from build123d import *

# Parameters (mm, degrees)
SKETCH2_W           = 42
SKETCH2_H           = 42
BOSS_EXTRUDE1_DEPTH = 100
SKETCH3_W           = 10.5
SKETCH3_H           = 42
BOSS_EXTRUDE2_DEPTH = 22
BOSS_EXTRUDE3_DEPTH = 10.5
BOSS_EXTRUDE4_START = -10.5
BOSS_EXTRUDE4_DEPTH = 10.5
SKETCH6_W           = 32
SKETCH6_H           = 32
CUT_EXTRUDE1_DEPTH  = 27
SKETCH7_R           = 3.95
CUT_EXTRUDE2_DEPTH  = 107.92637654
SKETCH9_R           = 3.95
CUT_EXTRUDE3_DEPTH  = 107.92637654
CUT_EXTRUDE4_DEPTH  = 21
FILLET1_R           = 5


with BuildPart() as part:
    # Sketch2 → Boss-Extrude1 (new body)
    with BuildSketch(Plane.XY):
        Rectangle(SKETCH2_W, SKETCH2_H)
    extrude(amount=BOSS_EXTRUDE1_DEPTH)

    # Sketch3 → Boss-Extrude2 (add)
    with BuildSketch(Plane(origin=(0, 0, 0), x_dir=(-1, 0, 0), z_dir=(0, 0, -1))):
        with Locations((15.75, 0)):
            Rectangle(SKETCH3_W, SKETCH3_H)
        with Locations((-15.75, 0)):
            Rectangle(SKETCH3_W, SKETCH3_H)
    extrude(amount=BOSS_EXTRUDE2_DEPTH)

    # Sketch4 → Boss-Extrude3 (add)
    with BuildSketch(Plane.ZY.offset(21)):
        with BuildLine():
            Line((-22, -21), (-22, 21))
            ThreePointArc((-22, 21), (-43, 0), (-22, -21))
        make_face()
    extrude(amount=-BOSS_EXTRUDE3_DEPTH)

    # Sketch5 → Boss-Extrude4 (add)
    with BuildSketch(Plane(origin=(21, 0, 0), x_dir=(0, 0, -1), z_dir=(1, 0, 0)).offset(BOSS_EXTRUDE4_START)):
        with BuildLine():
            Line((22, 21), (22, -21))
            ThreePointArc((22, -21), (43, 0), (22, 21))
        make_face()
    extrude(amount=BOSS_EXTRUDE4_DEPTH)

    # Sketch6 → Cut-Extrude1 (cut)
    with BuildSketch(Plane.XY.offset(100)):
        Rectangle(SKETCH6_W, SKETCH6_H)
    extrude(amount=-CUT_EXTRUDE1_DEPTH, mode=Mode.SUBTRACT)

    # Sketch7 → Cut-Extrude2 (cut, through all)
    with BuildSketch(Plane.ZY.offset(-10.5)):
        with Locations((-22, 0)):
            Circle(SKETCH7_R)
    extrude(amount=-CUT_EXTRUDE2_DEPTH, mode=Mode.SUBTRACT)

    # Sketch9 → Cut-Extrude3 (cut, through all)
    with BuildSketch(Plane(origin=(-10.5, 0, 0), x_dir=(0, 0, -1), z_dir=(1, 0, 0))):
        with Locations(Location((24, 0, 0), (0, 0, 90))):
            Circle(SKETCH9_R)
    extrude(amount=-CUT_EXTRUDE3_DEPTH, mode=Mode.SUBTRACT)

    # Sketch11 → Cut-Extrude4 (cut)
    with BuildSketch(Plane.ZY.offset(-10.5)):
        Polygon((0, 21), (0, 0), (29.025198915, 21), align=None)
        Polygon((29.025198915, -21), (0, 0), (0, -21), align=None)
    extrude(amount=CUT_EXTRUDE4_DEPTH, mode=Mode.SUBTRACT)

    # Fillet1
    fillet1_edges = [part.edges().sort_by_distance(p)[0] for p in [
        (0, 0, 0),
    ]]
    fillet(fillet1_edges, radius=FILLET1_R)


solid = part.part
For this review, take the finished solid that the model builds, in its own axes (mm). A direction names the side the tool comes from. Round coordinates to 2 decimals unless told otherwise and drop trailing zeros. Write each loop counter-clockwise with the first axis right and the second up, starting at its lowest first coordinate (ties: lowest second). Pieces come first, ordered by that corner, then holes. Notation, with made-up numbers: (-16, 25) - (33, 25) arc R14 ccw to (33, 42) - close; hole circle Ø7 at (-37, 40). An arc over 180 degrees is marked (long way). Write item = value, one per line. Start each with the question number.
1. Consider section D-D on x = 3. State the section outline as (y, z) points.
2. Wall thickness on L1, parallel to X at y = 11.5, z = -32; L2, parallel to Y at x = 12, z = 76; L3, parallel to Y at x = 15, z = -22: over which ranges is each line inside the solid? List them lowest first.
3. Consider section A-A on z = -4. State the section outline as (x, y) points, plus the area to 3 significant figures.
4. Consider section C-C on x = -14. State the section outline as (y, z) points, plus the area to 3 significant figures.
5. For pin 1 Ø1 at (x, y) = (-3, -2) entering from -Z; pin 2 Ø5 at (x, y) = (1.5, -15) entering from -Z; pin 3 Ø4 at (x, z) = (-10.5, -25.5) entering from -Y, all flat-tipped, find the tip position at first contact; note any pin that passes through.
6. For faces 1 (the face through (15.68, -1.51, -18.35)), 2 (the face through (0, -16, 87)), 3 (the face through (0.15, 12.41, 17.15)), list the 3-axis set-ups (+Z, -Z, +X, -X, +Y, -Y) from which the entire face can be reached by the end or side of a thin tool; tool diameter is ignored.
7. Consider section B-B on y = 0. State the section outline as (x, z) points, plus the area to 3 significant figures.
8. Draft analysis for pull direction Z (two halves, no side actions). For faces 4 (the face through (-0.15, 0.07, 3.53)), 5 (the face through (-15.676, -0.856, -27.856)), 6 (the face through (0, 0, 73)), 7 (the face through (-16, 0, 87)), state which applies: released by +Z, released by -Z, zero draft, split by the parting line, or undercut.
Evaluation:
q1.outline = (-21, 29.03) - (-4.05, 5.6) arc R5 ccw to (4.05, 5.6) - (21, 29.03) - (21, 100) - (16, 100) - (16, 73) - (-16, 73) - (-16, 100) - (-21, 100) - close
q2.L1 = -21 to -10.5, 10.5 to 21
q2.L2 = -21 to -16, 16 to 21
q2.L3 = -21 to -3.95, 3.95 to 21
q3.outline = (-21, -21) - (-10.5, -21) - (-10.5, 21) - (-21, 21) - close; (10.5, -21) - (21, -21) - (21, 21) - (10.5, 21) - close
q3.area = 882 mm2
q4.outline = (-21, -22) arc R21 ccw to (21, -22) - (21, 100) - (16, 100) - (16, 73) - (-16, 73) - (-16, 100) - (-21, 100) - close; hole circle Ø7.9 at (0, -24)
q4.area = 4,900 mm2
q5.pin_1 = 3.76
q5.pin_2 = 17.28
q5.pin_3 = -20.95
q6.face_1 = +X
q6.face_2 = +Z
q6.face_3 = -Z, +Y
q7.outline = (-21, -43) - (-10.5, -43) - (-10.5, -27.95) - (-21, -27.95) - close; (-21, -20.05) - (-10.5, -20.05) - (-10.5, 3.53) - (10.5, 3.53) - (10.5, -18.05) - (21, -18.05) - (21, 100) - (16, 100) - (16, 73) - (-16, 73) - (-16, 100) - (-21, 100) - close; (10.5, -43) - (21, -43) - (21, -25.95) - (10.5, -25.95) - close
q7.area = 4,000 mm2
q8.face_4 = released by -Z
q8.face_5 = undercut
q8.face_6 = released by +Z
q8.face_7 = zero draft
